Verification items for the finished model (mm, model axes). A direction names the side the tool comes from. Round coordinates to 2 decimals unless told otherwise and drop trailing zeros. Order: outer loops, then holes, each group sorted by start corner. A loop starts at its lowest first (then second) coordinate and runs counter-clockwise, first axis right, second up. Notation, with made-up numbers: (10.5, 34.25) -> (66.5, 34.25) arc R15 ccw to (66.5, 41.25) -> close; hole circle Ø11 at (6.25, 20). An arc over 180 degrees is marked (long way). Return JSON: item names as keys, results as strings. Group by question number.
1) Section check B-B on z = 7. Enter the section's corners in (x, y), plus the area to 3 significant figures.
2) Section check C-C on y = 29.5. Enter the section's corners in (x, z).
3) Section check A-A on x = -24. Enter the section's corners in (y, z), plus the area to 3 significant figures.
4) Tool access check on faces 1 (the flat face through (1, -51.438, 10)), 2 (the flat face through (15.742, 2, 11)). Record the directions out of +Z, -Z, +X, -X, +Y, -Y that give a thin tool (end or side, any length) a straight path to the whole face; none if there is none.
5) Scan lines: L1, parallel to X at y = -33, z = 11.25; L2, parallel to Y at x = 40, z = 4.5; L3, parallel to Z at x = -9.5, y = -1. Record each from-to range of solid material in increasing order.
6) Depth check by flat-ended pin: pin 1 (8 mm diameter, centred on x = -28, y = 17.5, fed in from +Z). Enter the tip coordinate at first touch or a pass-through.
7) Draft check along X on faces 3 (the flat face through (-17, 55.562, 11)), 4 (the flat face through (-48.258, 2, 10)), 5 (the flat face through (50.742, 2, 10)). Enter one of: pulls with the +X half, pulls with the -X half, needs draft (parallel to the pull), parting line crosses it, or undercut.
```python
from build123d import *

# Parameters (mm, degrees)
F0_W     = 99
F0_H     = 109
F1_DEPTH = 20
F2_T     = -2
F3_W     = 2
F3_H     = 105
F4_DEPTH = 18
F5_R     = 2


with BuildPart() as f1:
    # F0 (on Top) → F1 (new body)
    with BuildSketch(Plane.XY):
        with Locations((1.24195, 3.062002)):
            Rectangle(F0_W, F0_H)
    extrude(amount=F1_DEPTH)

    # F2
    f2_openings = [f1.faces().sort_by_distance(p)[0] for p in [
        (1.24195, 3.062002, 20),
    ]]
    offset(amount=F2_T, openings=f2_openings)

    # F3 (on face) → F4 (join, through all)
    with BuildSketch(Plane.XY.offset(2)):
        with Locations((14.74195, 3.062002)):
            Rectangle(F3_W, F3_H)
    extrude(amount=F4_DEPTH)

    # F5
    f5_edges = [f1.edges().sort_by_distance(p)[0] for p in [
        (-48.25805, 57.562002, 10),
        (-48.25805, -51.437998, 10),
        (50.74195, -51.437998, 10),
        (50.74195, 57.562002, 10),
    ]]
    fillet(f5_edges, radius=F5_R)


solid = f1.part
```
Check result:
{
 "1": {"outline": "(-48.26, -49.44) arc R2 ccw to (-46.26, -51.44) -> (48.74, -51.44) arc R2 ccw to (50.74, -49.44) -> (50.74, 55.56) arc R2 ccw to (48.74, 57.56) -> (-46.26, 57.56) arc R2 ccw to (-48.26, 55.56) -> close; hole (-46.26, -49.44) -> (13.74, -49.44) -> (13.74, 55.56) -> (-46.26, 55.56) -> close; hole (15.74, -49.44) -> (48.74, -49.44) -> (48.74, 55.56) -> (15.74, 55.56) -> close", "area": "1,020 mm^2"},
 "2": {"outline": "(-48.26, 0) -> (50.74, 0) -> (50.74, 20) -> (48.74, 20) -> (48.74, 2) -> (15.74, 2) -> (15.74, 20) -> (13.74, 20) -> (13.74, 2) -> (-46.26, 2) -> (-46.26, 20) -> (-48.26, 20) -> close"},
 "3": {"outline": "(-51.44, 0) -> (57.56, 0) -> (57.56, 20) -> (55.56, 20) -> (55.56, 2) -> (-49.44, 2) -> (-49.44, 20) -> (-51.44, 20) -> close", "area": "290 mm^2"},
 "4": {"face 1": "+Z, -Z, +X, -X, -Y", "face 2": "+Z"},
 "5": {"L1": "-48.26 to -46.26, 13.74 to 15.74, 48.74 to 50.74", "L2": "-51.44 to -49.44, 55.56 to 57.56", "L3": "0 to 2"},
 "6": {"pin 1": "z = 2"},
 "7": {"face 3": "undercut", "face 4": "pulls with the -X half", "face 5": "pulls with the +X half"}
}
